Geometry check sheet. Reference: the model listing, model coordinates, mm. A direction names the side the tool comes from. Give positions to 0.01 mm unless a question says otherwise; leave off trailing zeros. Loops run counter-clockwise (first coordinate to the right, second up) from the corner with the lowest first, then second, coordinate; pieces in that order, holes last. Notation, with made-up numbers: (7, 84) - (55, 84) arc R11 cw to (55, 104) - close; hole circle Ø10 at (33, -20). An arc over 180 degrees is marked (long way). Write item = value, one per line. Start each with the question number.
from build123d import *

# Parameters (mm, degrees)
SKETCH1_W           = 36
SKETCH1_H           = 36
BOSS_EXTRUDE1_DEPTH = 3
SKETCH2_R           = 1.5
CUT_EXTRUDE1_DEPTH  = 3
SKETCH3_W           = 6
SKETCH3_H           = 25
BOSS_EXTRUDE2_DEPTH = 70
CUT_EXTRUDE2_DEPTH  = 70
FILLET1_R           = 8
FILLET2_R           = 8
CUT_EXTRUDE3_DEPTH  = 2


with BuildPart() as part:
    # Sketch1 → Boss-Extrude1 (new body)
    with BuildSketch(Plane(origin=(0, 0, 0), x_dir=(1, 0, 0), z_dir=(0, 1, 0))):
        Rectangle(SKETCH1_W, SKETCH1_H)
    extrude(amount=BOSS_EXTRUDE1_DEPTH)

    # Sketch2 → Cut-Extrude1 (cut)
    with BuildSketch(Plane(origin=(0, 3, 0), x_dir=(1, 0, 0), z_dir=(0, 1, 0))):
        with Locations(Location((10, 0, 0), (0, 0, 270))):
            Circle(SKETCH2_R)
        with Locations(Location((-10, 0, 0), (0, 0, 270))):
            Circle(SKETCH2_R)
    extrude(amount=-CUT_EXTRUDE1_DEPTH, mode=Mode.SUBTRACT)

    # Sketch3 → Boss-Extrude2 (add)
    with BuildSketch(Plane(origin=(0, 3, 0), x_dir=(1, 0, 0), z_dir=(0, 1, 0))):
        Rectangle(SKETCH3_W, SKETCH3_H)
    extrude(amount=BOSS_EXTRUDE2_DEPTH)

    # Sketch4 → Cut-Extrude2 (cut)
    with BuildSketch(Plane(origin=(3, 0, 0), x_dir=(0, 0, -1), z_dir=(1, 0, 0))):
        with BuildLine():
            Line((-3, 28), (-3, 63))
            ThreePointArc((-3, 63), (0, 66), (3, 63))
            Line((3, 63), (3, 28))
            ThreePointArc((3, 28), (0, 25), (-3, 28))
        make_face()
    extrude(amount=-CUT_EXTRUDE2_DEPTH, mode=Mode.SUBTRACT)

    # Fillet1
    fillet1_edges = [part.edges().sort_by_distance(p)[0] for p in [
        (0, 73, -12.5),
    ]]
    fillet(fillet1_edges, radius=FILLET1_R)

    # Fillet2
    fillet2_edges = [part.edges().sort_by_distance(p)[0] for p in [
        (0, 73, 12.5),
    ]]
    fillet(fillet2_edges, radius=FILLET2_R)

    # Sketch5 → Cut-Extrude3 (cut)
    with BuildSketch(Plane(origin=(3, 0, 0), x_dir=(0, 0, -1), z_dir=(1, 0, 0))):
        with BuildLine():
            Line((4.5, 71), (-4.5, 71))
            ThreePointArc((-4.5, 71), (-8.742640687, 69.242640687), (-10.5, 65))
            Line((-10.5, 65), (-10.5, 5))
            Line((-10.5, 5), (10.5, 5))
            Line((10.5, 5), (10.5, 65))
            ThreePointArc((10.5, 65), (8.742640687, 69.242640687), (4.5, 71))
        make_face()
        with BuildLine():
            Line((5, 28), (5, 63))
            ThreePointArc((5, 63), (0, 68), (-5, 63))
            Line((-5, 63), (-5, 28))
            ThreePointArc((-5, 28), (0, 23), (5, 28))
        make_face(mode=Mode.SUBTRACT)
    extrude(amount=-CUT_EXTRUDE3_DEPTH, mode=Mode.SUBTRACT)


solid = part.part
1) Cross-section at B-B on y = 35. Enter the section's corners in (x, z), and give its area (3 significant figures).
2) Release check for a two-part mould opening along Z. For faces 1 (the face through (3, 45.2, -3.3)), 2 (the face through (0, 25, 0)), 3 (the face through (0, 34, -12.5)) record: pulls with the +Z half, pulls with the -Z half, needs draft (parallel to the pull), parting line crosses it, or undercut.
3) Gauge pin test, flat ends, axial feed: P1, Ø0.6, axis at x = 1.5, y = 43.5, coming from the +Z side; P2, Ø2, axis at x = 2, z = 5, coming from the +Y side; P3, Ø5, axis at x = 1, z = 12, coming from the +Y side (3 decimals); P4, Ø5, axis at x = 9.5, z = 5.5, coming from the +Y side. Record the tip position at first contact, or that the pin passes through.
4) Cross-section at D-D on x = 13. Enter the section's corners in (y, z), and give its area (3 significant figures).
5) Cross-section at C-C on z = 8. Enter the section's corners in (x, y), and give its area (3 significant figures).
6) Tool access check on faces 4 (the face through (-3, 38, -5)), 5 (the face through (0, 45, 3)), 6 (the face through (0, 1, -18)), 7 (the face through (2, 46, 5)), 8 (the face through (0, 0, 0)). Record the directions out of +Z, -Z, +X, -X, +Y, -Y that give a thin tool (end or side, any length) a straight path to the whole face; none if there is none.
7) Cross-section at A-A on x = -10. Enter the section's corners in (y, z).
8) Material ranges on line 1 along X through (y, z) = (1.05, 0); line 2 along Y through (x, z) = (14.5, 1.5); line 3 along X through (y, z) = (31, -8), recorded low to high.
Checked values:
q1.outline = (-3, -12.5) - (3, -12.5) - (3, -10.5) - (1, -10.5) - (1, -5) - (3, -5) - (3, -3) - (-3, -3) - close; (-3, 3) - (3, 3) - (3, 5) - (1, 5) - (1, 10.5) - (3, 10.5) - (3, 12.5) - (-3, 12.5) - close
q1.area = 92.0 mm²
q2.face_1 = needs draft
q2.face_2 = undercut
q2.face_3 = pulls with the -Z half
q3.P1 = 12.5
q3.P2 = 73
q3.P3 = 71.245
q3.P4 = 3
q4.outline = (0, -18) - (3, -18) - (3, 18) - (0, 18) - close
q4.area = 108 mm²
q5.outline = (-18, 0) - (18, 0) - (18, 3) - (3, 3) - (3, 5) - (1, 5) - (1, 69.87) - (3, 69.87) - (3, 72.19) - (-3, 72.19) - (-3, 3) - (-18, 3) - close
q5.area = 393 mm²
q6.face_4 = +Z, -Z, -X, +Y
q6.face_5 = +X, -X
q6.face_6 = -Z, +X, -X, +Y, -Y
q6.face_7 = +X
q6.face_8 = +Z, -Z, +X, -X, -Y
q7.outline = (0, -18) - (3, -18) - (3, -1.5) - (0, -1.5) - close; (0, 1.5) - (3, 1.5) - (3, 18) - (0, 18) - close
q8.line_1 = -18 to -11.5, -8.5 to 8.5, 11.5 to 18
q8.line_2 = 0 to 3
q8.line_3 = -3 to 1
